Design review of the part built by this model. Coordinates are the model's own, in mm. Face numbers are marked on the shaded views. A direction names the side the tool comes from. Round coordinates to 2 decimals unless told otherwise and drop trailing zeros. Order: outer loops, then holes, each group sorted by start corner. A loop starts at its lowest first (then second) coordinate and runs counter-clockwise, first axis right, second up. Notation, with made-up numbers: (53, 55.25) - (82, 55.25) arc R24 cw to (82, 67.25) - close; hole circle Ø9 at (-17.5, 54). An arc over 180 degrees is marked (long way). Write item = value, one per line.
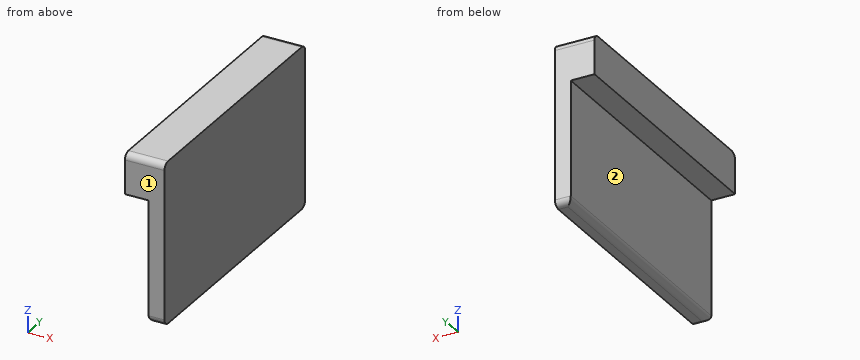
from build123d import *

# Parameters (mm, degrees)
SKETCH1_W           = 7.5
SKETCH1_H           = 12.7
BOSS_EXTRUDE1_DEPTH = 79.375
FILLET1_R           = 2


with BuildPart() as part:
    # Sketch1 → Boss-Extrude1 (new body)
    with BuildSketch(Plane(origin=(0, 0, 0), x_dir=(1, 0, 0), z_dir=(0, 1, 0))):
        with Locations((3.75, 6.35)):
            Rectangle(SKETCH1_W, SKETCH1_H)
        Polygon((7.5, 12.7), (7.5, 0), (12.5, 0), (12.5, 50.8), (7.5, 50.8), align=None)
    extrude(amount=BOSS_EXTRUDE1_DEPTH)

    # Fillet1
    fillet1_edges = [part.edges().sort_by_distance(p)[0] for p in [
        (6.25, 0, 0),
        (7.5, 39.6875, -50.8),
        (10, 79.375, -50.8),
        (6.25, 79.375, 0),
        (10, 0, -50.8),
    ]]
    fillet(fillet1_edges, radius=FILLET1_R)


solid = part.part
1) We need section A-A on y = 24. Write out the cut boundary in (x, z).
Findings:
outline = (0, -12.7) - (7.5, -12.7) - (7.5, -48.8) arc R2 ccw to (9.5, -50.8) - (12.5, -50.8) - (12.5, 0) - (0, 0) - close
2) We need section B-B on x = 1.5. Write out the cut boundary in (y, z) (3 decimals).
Findings:
outline = (0, -12.7) - (79.375, -12.7) - (79.375, -2) arc R2 ccw to (77.375, 0) - (2, 0) arc R2 ccw to (0, -2) - close
3) Clearance check with flat-ended pins moving along their axes: pin 1 Ø1 at (x, y) = (3.5, 25.5) entering from -Z; pin 2 Ø11 at (y, z) = (44, -32.5) entering from -X. State where each tip first meets the part, or that it passes through.
Findings:
pin_1 = -12.7
pin_2 = 7.5
4) We need section C-C on z = -44. Write out the cut boundary in (x, y) (3 decimals), and give its area (3 significant figures).
Findings:
outline = (7.5, 0) - (12.5, 0) - (12.5, 79.375) - (7.5, 79.375) - close
area = 397 mm^2
5) For the marked faces 1 and 2, list the 3-axis set-ups (+Z, -Z, +X, -X, +Y, -Y) from which the entire face can be reached by the end or side of a thin tool; tool diameter is ignored.
Findings:
face_1 = +Z, -Z, +X, -X, -Y
face_2 = -Z, -X, +Y, -Y
6) To check wall thickness, follow L1, parallel to X at y = 73, z = -39; L2, parallel to Z at x = 4.5, y = 21; L3, parallel to Z at x = 8.5, y = 36. State the ranges of each line that lie inside material, in increasing order. Write a range as from..to.
Findings:
L1 = 7.5..12.5
L2 = -12.7..0
L3 = -50.53..0
